Autodesk Inventor part; units mm, degrees
ref_plane "ANBAU_XY" through (0, 0, -278) normal (0, 1, 0) x (1, 0, 0)
ref_plane "ANBAU_YZ" through (0, 0, -278) normal (1, 0, 0) x (0, 0, -1)
ref_plane "ANBAU_ZX" through (0, 0, -278) normal (0, 0, -1) x (0, 1, 0)
sketch "Sketch_1" plane through (0, 0, 0) normal (0, 1, 0) x (-1, 0, 0)
  line L0 (72.5, -155.8931) -> (72.5, -6.7735)
  arc A0 (72.5, -6.7735) -> (70.7696, -4.7917) centre (70.5, -6.7735) ccw
  arc A1 (70.7696, -4.7917) -> (-70.7696, -4.7917) centre (0, -525) ccw
  arc A2 (-70.7696, -4.7917) -> (-72.5, -6.7735) centre (-70.5, -6.7735) ccw
  line L1 (-72.5, -6.7735) -> (-72.5, -155.8931)
  arc A3 (-72.5, -155.8931) -> (-72.408, -156.4104) centre (-71, -155.8931) ccw
  arc A4 (-72.408, -211.5896) -> (-72.408, -156.4104) centre (-147.5, -184) ccw
  arc A5 (-72.408, -211.5896) -> (-72.5, -212.1069) centre (-71, -212.1069) ccw
  line L2 (-72.5, -212.1069) -> (-72.5, -341.2265)
  arc A6 (-72.5, -341.2265) -> (-70.7696, -343.2083) centre (-70.5, -341.2265) ccw
  arc A7 (-70.7696, -343.2083) -> (70.7696, -343.2083) centre (0, 177) ccw
  arc A8 (70.7696, -343.2083) -> (72.5, -341.2265) centre (70.5, -341.2265) ccw
  line L3 (72.5, -341.2265) -> (72.5, -212.1069)
  arc A9 (72.5, -212.1069) -> (72.408, -211.5896) centre (71, -212.1069) ccw
  arc A10 (72.408, -156.4104) -> (72.408, -211.5896) centre (147.5, -184) ccw
  arc A11 (72.408, -156.4104) -> (72.5, -155.8931) centre (71, -155.8931) ccw
extrude "Extrusion1" add sketch "Sketch_1" along normal blind 50
sketch "Sketch_12" plane through (0, 0, 0) normal (0, 1, 0) x (-1, 0, 0)
  arc A0 (20.3731, -115.3216) -> (-20.3731, -115.3216) centre (0, -90) ccw
  arc A1 (-20, -116.1008) -> (-20.3731, -115.3216) centre (-21, -116.1008) ccw
  line L0 (-20, -116.1008) -> (-20, -290.5)
  arc A2 (-20, -290.5) -> (20, -290.5) centre (0, -290.5) ccw
  line L1 (20, -290.5) -> (20, -116.1008)
  arc A3 (20.3731, -115.3216) -> (20, -116.1008) centre (21, -116.1008) ccw
extrude "Extrusion2" cut sketch "Sketch_12" along normal blind 41
sketch "Sketch_2" plane through (0, 0, 0) normal (0, 1, 0) x (-1, 0, 0)
  circle A0 centre (0, -278) radius 32.5
extrude "Extrusion3" cut sketch "Sketch_2" along normal blind 23
sketch "Sketch_3" plane through (0, 0, 0) normal (0, 1, 0) x (-1, 0, 0)
  circle A0 centre (0, -278) radius 20
extrude "Extrusion4" cut sketch "Sketch_3" along normal blind 45
sketch "Sketch_4" plane through (0, 0, 0) normal (0, 1, 0) x (-1, 0, 0)
  circle A0 centre (0, -90) radius 20
extrude "Extrusion5" cut sketch "Sketch_4" along normal blind 45
sketch "Sketch_21" plane through (0, 0, 0) normal (0, 1, 0) x (-1, 0, 0)
  arc A0 (50.0467, -105.8611) -> (-50.0467, -105.8611) centre (0, -90) ccw
  arc A1 (-50, -106.1632) -> (-50.0467, -105.8611) centre (-51, -106.1632) ccw
  line L0 (-50, -106.1632) -> (-50, -261.8368)
  arc A2 (-50.0467, -262.1389) -> (-50, -261.8368) centre (-51, -261.8368) ccw
  arc A3 (-50.0467, -262.1389) -> (50.0467, -262.1389) centre (0, -278) ccw
  arc A4 (50, -261.8368) -> (50.0467, -262.1389) centre (51, -261.8368) ccw
  line L1 (50, -261.8368) -> (50, -106.1632)
  arc A5 (50.0467, -105.8611) -> (50, -106.1632) centre (51, -106.1632) ccw
extrude "Extrusion6" cut sketch "Sketch_21" along normal blind 5
sketch "Sketch7" plane through (0, 50, 0) normal (0, 1, 0) x (1, 0, 0)
  point P0 (0, 15)
hole "Hole1" at (0, 50, -15) direction (0, -1, 0) diameter 9 depth 50 counterbore diameter 15 counterbore depth 9
sketch "Sketch8" plane through (0, 50, 0) normal (0, 1, 0) x (1, 0, 0)
  point P0 (57.5, 208)
hole "Hole2" at (57.5, 50, -208) direction (0, -1, 0) diameter 9 depth 50 counterbore diameter 15 counterbore depth 9
sketch "Sketch9" plane through (0, 50, 0) normal (0, 1, 0) x (1, 0, 0)
  point P0 (57.5, 313)
hole "Hole3" at (57.5, 50, -313) direction (0, -1, 0) diameter 9 depth 50 counterbore diameter 15 counterbore depth 9
sketch "Sketch10" plane through (0, 50, 0) normal (0, 1, 0) x (1, 0, 0)
  point P0 (57.5, 78)
hole "Hole4" at (57.5, 50, -78) direction (0, -1, 0) diameter 9 depth 50 counterbore diameter 15 counterbore depth 9
sketch "Sketch11" plane through (0, 50, 0) normal (0, 1, 0) x (1, 0, 0)
  point P0 (-57.5, 208)
hole "Hole5" at (-57.5, 50, -208) direction (0, -1, 0) diameter 9 depth 50 counterbore diameter 15 counterbore depth 9
sketch "Sketch12" plane through (0, 50, 0) normal (0, 1, 0) x (1, 0, 0)
  point P0 (-57.5, 313)
hole "Hole6" at (-57.5, 50, -313) direction (0, -1, 0) diameter 9 depth 50 counterbore diameter 15 counterbore depth 9
sketch "Sketch13" plane through (0, 50, 0) normal (0, 1, 0) x (1, 0, 0)
  point P0 (-57.5, 78)
hole "Hole7" at (-57.5, 50, -78) direction (0, -1, 0) diameter 9 depth 50 counterbore diameter 15 counterbore depth 9
sketch "Sketch14" plane through (0, 50, 0) normal (0, 1, 0) x (1, 0, 0)
  point P0 (44.5, 322.5)
hole "Hole8" at (44.5, 50, -322.5) direction (0, -1, 0) diameter 8.376 depth 30 tip angle 120 countersink diameter 10 countersink angle 90
sketch "Sketch15" plane through (0, 50, 0) normal (0, 1, 0) x (1, 0, 0)
  point P0 (-44.5, 322.5)
hole "Hole9" at (-44.5, 50, -322.5) direction (0, -1, 0) diameter 8.376 depth 30 tip angle 120 countersink diameter 10 countersink angle 90
sketch "Sketch16" plane through (0, 50, 0) normal (0, 1, 0) x (1, 0, 0)
  point P0 (44.5, 233.5)
hole "Hole10" at (44.5, 50, -233.5) direction (0, -1, 0) diameter 8.376 depth 30 tip angle 120 countersink diameter 10 countersink angle 90
sketch "Sketch17" plane through (0, 50, 0) normal (0, 1, 0) x (1, 0, 0)
  point P0 (-44.5, 233.5)
hole "Hole11" at (-44.5, 50, -233.5) direction (0, -1, 0) diameter 8.376 depth 30 tip angle 120 countersink diameter 10 countersink angle 90
ref_plane "ANBAU_XY" through (0, 0, -278) normal (0, 1, 0) x (1, 0, 0)
ref_plane "ANBAU_YZ" through (0, 0, -278) normal (1, 0, 0) x (0, 0, -1)
ref_plane "ANBAU_ZX" through (0, 0, -278) normal (0, 0, -1) x (0, 1, 0)
ref_plane "S1_1_XY" through (57.5, 41, -313) normal (0, 1, 0) x (1, 0, 0)
ref_plane "S1_1_YZ" through (57.5, 41, -313) normal (1, 0, 0) x (0, 0, -1)
ref_plane "S1_1_ZX" through (57.5, 41, -313) normal (0, 0, -1) x (0, 1, 0)
ref_plane "S1_2_XY" through (57.5, 41, -208) normal (0, 1, 0) x (1, 0, 0)
ref_plane "S1_2_YZ" through (57.5, 41, -208) normal (1, 0, 0) x (0, 0, -1)
ref_plane "S1_2_ZX" through (57.5, 41, -208) normal (0, 0, -1) x (0, 1, 0)
ref_plane "S1_3_XY" through (57.5, 41, -78) normal (0, 1, 0) x (1, 0, 0)
ref_plane "S1_3_YZ" through (57.5, 41, -78) normal (1, 0, 0) x (0, 0, -1)
ref_plane "S1_3_ZX" through (57.5, 41, -78) normal (0, 0, -1) x (0, 1, 0)
ref_plane "S2_1_XY" through (-57.5, 41, -313) normal (0, 1, 0) x (1, 0, 0)
ref_plane "S2_1_YZ" through (-57.5, 41, -313) normal (1, 0, 0) x (0, 0, -1)
ref_plane "S2_1_ZX" through (-57.5, 41, -313) normal (0, 0, -1) x (0, 1, 0)
ref_plane "S2_2_XY" through (-57.5, 41, -208) normal (0, 1, 0) x (1, 0, 0)
ref_plane "S2_2_YZ" through (-57.5, 41, -208) normal (1, 0, 0) x (0, 0, -1)
ref_plane "S2_2_ZX" through (-57.5, 41, -208) normal (0, 0, -1) x (0, 1, 0)
ref_plane "S2_3_XY" through (-57.5, 41, -78) normal (0, 1, 0) x (1, 0, 0)
ref_plane "S2_3_YZ" through (-57.5, 41, -78) normal (1, 0, 0) x (0, 0, -1)
ref_plane "S2_3_ZX" through (-57.5, 41, -78) normal (0, 0, -1) x (0, 1, 0)
ref_plane "S3_XY" through (0, 41, -15) normal (0, 1, 0) x (1, 0, 0)
ref_plane "S3_YZ" through (0, 41, -15) normal (1, 0, 0) x (0, 0, -1)
ref_plane "S3_ZX" through (0, 41, -15) normal (0, 0, -1) x (0, 1, 0)
properties part number "1464690 EAMM-U-145-D100-...-348S---(OT)"
Geometry check sheet. Reference: the model listing, model coordinates, mm. A direction names the side the tool comes from. Give positions to 0.01 mm unless a question says otherwise; leave off trailing zeros. Order: outer loops, then holes, each group sorted by start corner. A loop starts at its lowest first (then second) coordinate and runs counter-clockwise, first axis right, second up.
1) Tool access check on faces 5 (the flat face through (20, 23, -202)), 6 (the cylindrical face through (-59.753, 45.437, -200.846)), 7 (the cylindrical face through (59.22, 20.21, -308.84)). Record the directions out of +Z, -Z, +X, -X, +Y, -Y that give a thin tool (end or side, any length) a straight path to the whole face; none if there is none.
Results are:
face 5: -Y
face 6: +Y
face 7: +Y, -Y
2) Cross-section at A-A (z = -15). Record the boundary of the cut face in (x, y).
Results are:
outline: (-72.5, 0) - (-4.5, 0) - (-4.5, 41) - (-7.5, 41) - (-7.5, 50) - (-72.5, 50) - close; (4.5, 0) - (72.5, 0) - (72.5, 50) - (7.5, 50) - (7.5, 41) - (4.5, 41) - close
3) Cross-section at D-D (x = -26). Record the boundary of the cut face in (y, z), then the cut area to 3 significant figures.
Results are:
outline: (0, -347.36) - (50, -347.36) - (50, -0.64) - (0, -0.64) - (0, -44.39) - (5, -44.39) - (5, -70.5) - (41, -70.5) - (41, -109.5) - (5, -109.5) - (5, -258.5) - (23, -258.5) - (23, -297.5) - (5, -297.5) - (5, -323.61) - (0, -323.61) - close
area: 13,800 mm2
4) Draft check along Z on faces 1 (the cylindrical face through (-1, 25, -348)), 2 (the flat face through (62.4, 41, -78.1)), 3 (the cylindrical face through (1, 25, 0)), 4 (the cylindrical face through (1.12, 22.75, -57.52)). Enter one of: released by +Z, released by -Z, zero draft, split by the parting line, or undercut.
Results are:
face 1: released by -Z
face 2: undercut
face 3: released by +Z
face 4: undercut
5) Cross-section at C-C (x = 12). Record the boundary of the cut face in (y, z), then the cut area to 3 significant figures.
Results are:
outline: (0, -347.86) - (50, -347.86) - (50, -0.14) - (0, -0.14) - (0, -38.89) - (5, -38.89) - (5, -59.8) - (41, -59.8) - (41, -74) - (45, -74) - (45, -106) - (41, -106) - (41, -262) - (45, -262) - (45, -294) - (41, -294) - (41, -306.5) - (23, -306.5) - (23, -308.2) - (5, -308.2) - (5, -329.11) - (0, -329.11) - close
area: 6,770 mm2
6) Gauge pin test, flat ends, axial feed: pin 1 (1 mm diameter, centred on x = -50.5, y = 44.5, fed in from -Z); pin 2 (20 mm diameter, centred on x = -10, z = -88.5, fed in from -Y); pin 3 (10.5 mm diameter, centred on x = 0, z = -15, fed in from +Y). Record the tip position at first contact, or that the pin passes through.
Results are:
pin 1: stops at z = -345.61
pin 2: stops at y = 41
pin 3: stops at y = 41
7) Material ranges on probe 1 along X at (y, z) = (32, -322.5); probe 2 along X at (y, z) = (45, -313); probe 3 along X at (y, z) = (26, -233), recorded low to high.
Results are:
probe 1: x = -72.5 to -48.69, -40.31 to 40.31, 48.69 to 72.5
probe 2: x = -72.5 to -65, -50 to 50, 65 to 72.5
probe 3: x = -72.5 to -48.66, -40.34 to -20, 20 to 40.34, 48.66 to 72.5
8) Cross-section at B-B (z = -208). Record the boundary of the cut face in (x, y).
Results are:
outline: (-71.18, 0) - (-62, 0) - (-62, 41) - (-65, 41) - (-65, 50) - (-71.18, 50) - close; (-53, 0) - (-50, 0) - (-50, 5) - (-20, 5) - (-20, 41) - (20, 41) - (20, 5) - (50, 5) - (50, 0) - (53, 0) - (53, 41) - (50, 41) - (50, 50) - (-50, 50) - (-50, 41) - (-53, 41) - close; (62, 0) - (71.18, 0) - (71.18, 50) - (65, 50) - (65, 41) - (62, 41) - close
